Design review of the part built by this model. Coordinates are the model's own, in mm. Round coordinates to 2 decimals unless told otherwise and drop trailing zeros. Loops run counter-clockwise (first coordinate to the right, second up) from the corner with the lowest first, then second, coordinate; pieces in that order, holes last. Notation, with made-up numbers: M -8.5,78 L 40.5,78 A27 cw 40.5,103 Z; hole C 43.25,44.25 d11. An arc over 180 degrees is marked long. One line per item, written item: value. Start each with the question number.
Item 1: For line 1 along Z through (x, y) = (-2, 5.25); line 2 along X through (y, z) = (-1.25, 153); line 3 along Y through (x, z) = (-6, 269), list the stretches that pass through material, from the lowest coordinate up.
Item 2: We need section A-A (y = 0). Write out the cut boundary in (x, z).
Item 3: We need section B-B (z = 75.5). Write out the cut boundary in (x, y).
Item 4: Clearance check with a flat-ended pin moving along its axis: pin 1 (6 mm diameter, centred on x = -2, y = 3.5, fed in from -Z). State where the tip first meets the part, or that it passes through.
Autodesk Inventor part; units mm, degrees
ref_plane "YZ Plane" through (0, 0, 0) normal (1, 0, 0) x (0, 1, 0)
ref_plane "XZ Plane" through (0, 0, 0) normal (0, 1, 0) x (-1, 0, 0)
ref_plane "XY Plane" through (0, 0, 0) normal (0, 0, 1) x (1, 0, 0)
sketch "Sketch1" plane through (0, 0, 0) normal (0, 0, 1) x (1, 0, 0)
  line L0 (-7.2, -8.1) -> (7.2, -8.1)
  line L1 (7.2, -8.1) -> (7.2, 8.1)
  line L2 (7.2, 8.1) -> (-7.2, 8.1)
  line L3 (-7.2, 8.1) -> (-7.2, -8.1)
  line L4 (-6.2, 7.1) -> (6.2, 7.1)
  line L5 (6.2, 7.1) -> (6.2, -7.1)
  line L6 (6.2, -7.1) -> (-6.2, -7.1)
  line L7 (-6.2, -7.1) -> (-6.2, 7.1)
  dimension "d9" = 1
extrude "Extrusion2" add sketch "Sketch1" along normal blind 340
sketch "Sketch2" plane through (0, 0, 340) normal (0, 0, 1) x (1, 0, 0)
  line L0 (-7.2, -8.1) -> (7.2, -8.1) construction
  line L1 (-7.2, 8.1) -> (7.2, 8.1)
  line L2 (7.2, 8.1) -> (7.2, -8.1)
  line L3 (7.2, -8.1) -> (-7.2, -8.1)
  line L4 (-7.2, -8.1) -> (-7.2, 8.1)
  point P0 (0, 0)
extrude "Extrusion3" add sketch "Sketch2" against normal blind 2
sketch "Sketch3" plane through (0, 0, 0) normal (0, 0, -1) x (-1, 0, 0)
  line L0 (-7.2, -8.1) -> (-7.2, 8.1) construction
  line L1 (7.2, 8.1) -> (7.2, -8.1) construction
  line L2 (-7.2, -8.1) -> (7.2, -8.1)
  line L3 (7.2, -8.1) -> (7.2, 8.1)
  line L4 (7.2, 8.1) -> (-7.2, 8.1)
  line L5 (-7.2, 8.1) -> (-7.2, -8.1)
  point P0 (0, 0)
extrude "Extrusion4" add sketch "Sketch3" against normal blind 2
properties part number "PL_rod_single"
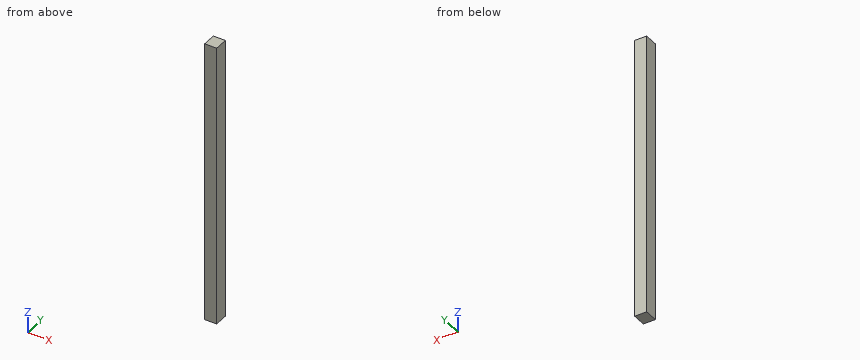
A:
1. line 1: 0 to 2, 338 to 340
1. line 2: -7.2 to -6.2, 6.2 to 7.2
1. line 3: -8.1 to -7.1, 7.1 to 8.1
2. outline: M -7.2,0 L 7.2,0 L 7.2,340 L -7.2,340 Z; hole M -6.2,2 L 6.2,2 L 6.2,338 L -6.2,338 Z
3. outline: M -7.2,-8.1 L 7.2,-8.1 L 7.2,8.1 L -7.2,8.1 Z; hole M -6.2,-7.1 L 6.2,-7.1 L 6.2,7.1 L -6.2,7.1 Z
4. pin 1: z = 0
